Input: part model. Units: mm. Frame: model coordinates. Give positions to 0.01 mm unless a question says otherwise; leave off trailing zeros. Order: outer loops, then holes, each group sorted by start corner. A loop starts at its lowest first (then second) coordinate and runs counter-clockwise, first axis right, second up. Notation, with made-up numbers: (-9, 85.25) - (26, 85.25) arc R12 cw to (26, 99.25) - close; hole circle Ø4 at (-38, 3.25). An arc over 180 degrees is marked (long way). Answer in a Markdown table with one row per item. Add a question column.
1. Mould query, pull axis Y, two halves, no side actions, for faces 1 (the face through (-30.38, -19.19, 3.45)), 2 (the face through (12.92, -19.19, 3.45)), 3 (the face through (34.4, -20.4, 3.5)), 4 (the face through (8, -9, 0)). Classes: released by +Y, released by -Y, zero draft, split by the parting line, or undercut.
2. Section query B-B on y = 25. Return loops of the section in (x, z).
3. Section query A-A on y = -12.5. Return loops of the section in (x, z).
4. Section query D-D on z = 2.25. Count the separate pieces of the cut face and the enclosed holes in it, and give its area (3 significant figures).
5. Contact query for flat-ended pins moving along their axis: pin 1 (4 mm diameter, centred on y = -8, z = 5, fed in from +X); pin 2 (1 mm diameter, centred on x = -16.5, z = 4, fed in from -Y); pin 3 (2 mm diameter, centred on y = 20.5, z = 5, fed in from +X). Output: stop coordinate, or through.
6. Section query C-C on x = 31.5. Return loops of the section in (y, z), and give its area (3 significant figures).
7. Ray query, line 1 (X direction, y = -13, z = 4.25); line 2 (Y direction, x = 0, z = 2); line 3 (Y direction, x = 13.5, z = 4). Return the intervals inside material, ascending. Write a range as [from, to].
```python
from build123d import *

# Parameters (mm, degrees)
F0_R     = 11
F1_DEPTH = 7
F2_R     = 9.999


# Not quite as in the source:
# - a fillet or chamfer is up to 0.001 mm smaller than in the source, because OpenCascade refuses the exact size


with BuildPart() as f1:
    # F0 (on Top) → F1 (new body)
    with BuildSketch(Plane.XY):
        with BuildLine():
            ThreePointArc((8.2915619759, 12.5), (0, 40), (-8.2915619759, 12.5))
            ThreePointArc((-8.2915619759, 12.5), (-12.9903810568, 7.5), (-14.9710985352, 0.9307033082))
            ThreePointArc((-14.9710985352, 0.9307033082), (-34.6410161514, -20), (-6.6795365594, -13.4307033082))
            ThreePointArc((-6.6795365594, -13.4307033082), (0, -15), (6.6795365594, -13.4307033082))
            ThreePointArc((6.6795365594, -13.4307033082), (34.6410161514, -20), (14.9710985352, 0.9307033082))
            ThreePointArc((14.9710985352, 0.9307033082), (12.9903810568, 7.5), (8.2915619759, 12.5))
        make_face()
        with Locations((-21.6506350946, -12.5)):
            Circle(F0_R, mode=Mode.SUBTRACT)
        with Locations((21.6506350946, -12.5)):
            Circle(F0_R, mode=Mode.SUBTRACT)
        Circle(F0_R, mode=Mode.SUBTRACT)
        with Locations((0, 25)):
            Circle(F0_R, mode=Mode.SUBTRACT)
    extrude(amount=F1_DEPTH)

    # F2 (radius 10 in the source; OpenCascade refuses exactly that, so slightly less here)
    f2_edges = [f1.edges().sort_by_distance(p)[0] for p in [
        (-8.291562, 12.5, 3.5),
        (-14.971099, 0.930703, 3.5),
        (-6.679537, -13.430703, 3.5),
        (6.679537, -13.430703, 3.5),
        (14.971099, 0.930703, 3.5),
        (8.291562, 12.5, 3.5),
    ]]
    fillet(f2_edges, radius=F2_R)


solid = f1.part
```
Answer:
| question | item | result |
|---|---|---|
| 1 | face 1 | undercut |
| 1 | face 2 | undercut |
| 1 | face 3 | split by the parting line |
| 1 | face 4 | zero draft |
| 2 | outline | (-15, 0) - (-11, 0) - (-11, 7) - (-15, 7) - close; (11, 0) - (15, 0) - (15, 7) - (11, 7) - close |
| 3 | outline | (-36.65, 0) - (-32.65, 0) - (-32.65, 7) - (-36.65, 7) - close; (-10.65, 0) - (10.65, 0) - (10.65, 7) - (-10.65, 7) - close; (32.65, 0) - (36.65, 0) - (36.65, 7) - (32.65, 7) - close |
| 4 | separate pieces | 1 |
| 4 | enclosed holes | 4 |
| 4 | area | 1,200 mm² |
| 5 | pin 1 | stops at x = 36.44 |
| 5 | pin 2 | stops at y = -26.76 |
| 5 | pin 3 | stops at x = 14.59 |
| 6 | outline | (-23.81, 0) - (-17.4, 0) - (-17.4, 7) - (-23.81, 7) - close; (-7.6, 0) - (-1.19, 0) - (-1.19, 7) - (-7.6, 7) - close |
| 6 | area | 89.8 mm² |
| 7 | line 1 | x = [-36.64, -32.64], [-10.66, 10.66], [32.64, 36.64] |
| 7 | line 2 | y = [-15, -11], [11, 14], [36, 40] |
| 7 | line 3 | y = [-25.09, -19.89], [-5.11, 6.71], [18.46, 31.54] |
